For this review, take the finished solid that the model builds, in its own axes (mm). Face numbers are marked on the shaded views. A direction names the side the tool comes from. Give positions to 0.01 mm unless a question says otherwise; leave off trailing zeros. Order: outer loops, then holes, each group sorted by start corner. A loop starts at its lowest first (then second) coordinate and runs counter-clockwise, first axis right, second up. Notation, with made-up numbers: M 18,-4.75 L 56,-4.75 A31 cw 56,19.25 Z; hole C -26.5,-37.75 d10. An arc over 180 degrees is marked long. Answer as CSV lines item,"result". Start each with the question number.
1. Clearance check with a flat-ended pin moving along its axis: P1, Ø12, axis at x = -8, y = 14, coming from the +Z side. State where the tip first meets the part, or that it passes through.
2. Mouldability with a two-part tool opening along Y and no side actions: class the marked faces 3, 4, 5 and 6 as pulls with the +Y half, pulls with the -Y half, needs draft (parallel to the pull), parting line crosses it, or undercut.
3. We need section B-B, the plane x = -11. Give the boundary of the cut face in (y, z), and give its area (3 significant figures).
4. We need section D-D, the plane z = 196. Give the boundary of the cut face in (x, y), and give its area (3 significant figures).
5. We need section A-A, the plane y = 10. Give the boundary of the cut face in (x, z), and give its area (3 significant figures).
6. For line 1 along X through (y, z) = (20.5, 45); line 2 along Y through (x, z) = (-7, 251.5), list the stretches that pass through material, from the lowest coordinate up.
7. Machinability: for the marked faces 1 and 2, which of the approach directions +Z, -Z, +X, -X, +Y, -Y give a long, thin tool a straight path to every point of the face, cutting with its end or side? Answer none if there is none.
8. We need section C-C, the plane z = 261. Give the boundary of the cut face in (x, y), and give its area (3 significant figures).
from build123d import *

# Parameters (mm, degrees)
F0_W     = 50
F0_H     = 50
F0_W_2   = 44.5
F0_H_2   = 44.5
F1_DEPTH = 300
F3_DEPTH = 30


with BuildPart() as f1:
    # F0 (on Top) → F1 (new body)
    with BuildSketch(Plane.XY):
        Rectangle(F0_W, F0_H)
        Rectangle(F0_W_2, F0_H_2, mode=Mode.SUBTRACT)
    extrude(amount=F1_DEPTH)

    # F2 (on Right) → F3 (cut, symmetric)
    with BuildSketch(Plane.YZ):
        Polygon((25, 300), (-25, 300), (25, 250), align=None)
    extrude(amount=F3_DEPTH, both=True, mode=Mode.SUBTRACT)


solid = f1.part
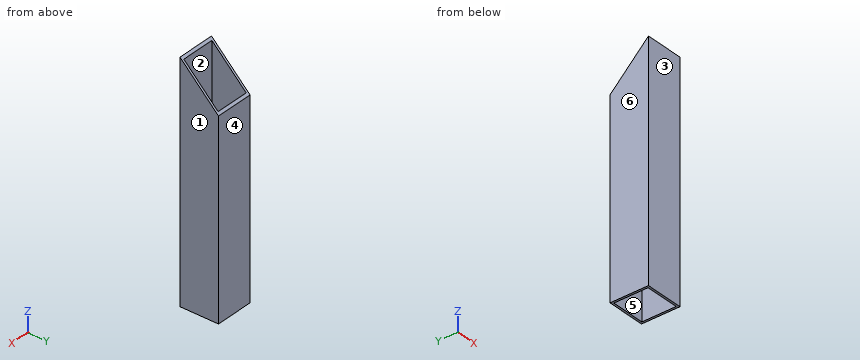
Result set:
1,P1,"through"
2,face 3,"pulls with the -Y half"
2,face 4,"pulls with the +Y half"
2,face 5,"undercut"
2,face 6,"needs draft"
3,outline,"M -25,0 L -22.25,0 L -22.25,297.25 L -25,300 Z; M 22.25,0 L 25,0 L 25,250 L 22.25,252.75 Z"
3,area,"1,510 mm2"
4,outline,"M -25,-25 L 25,-25 L 25,25 L -25,25 Z; hole M -22.25,-22.25 L 22.25,-22.25 L 22.25,22.25 L -22.25,22.25 Z"
4,area,"520 mm2"
5,outline,"M -25,0 L -22.25,0 L -22.25,265 L -25,265 Z; M 22.25,0 L 25,0 L 25,265 L 22.25,265 Z"
5,area,"1,460 mm2"
6,line 1,"-25 to -22.25, 22.25 to 25"
6,line 2,"-25 to -22.25, 22.25 to 23.5"
7,face 1,"+Z, -Z, +X, +Y, -Y"
7,face 2,"+Z, -Z"
8,outline,"M -25,-25 L 25,-25 L 25,14 L 22.25,14 L 22.25,-22.25 L -22.25,-22.25 L -22.25,14 L -25,14 Z"
8,area,"337 mm2"
